Source: three-view drawing plus pictorial views. Frame: mm from the lowest corner of the part. A direction names the side the tool comes from. Give positions to 0.01 mm unless a question says otherwise; leave off trailing zeros. Loops run counter-clockwise (first coordinate to the right, second up) from the corner with the lowest first, then second, coordinate; pieces in that order, holes last. Notation, with made-up numbers: M -36,83.25 L -29,83.25 A18 ccw -29,114.25 Z; hole C 28.5,52.25 d8. An arc over 180 degrees is marked long. Write item = value, one per line.
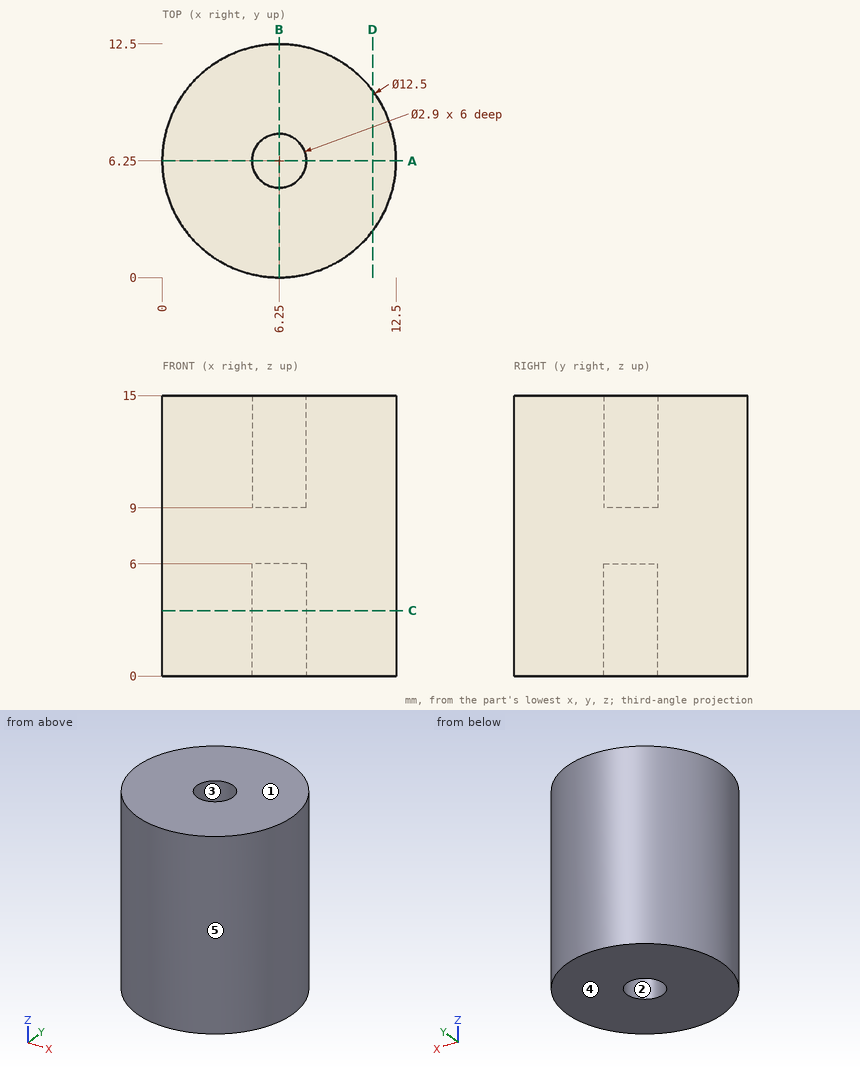
1. Cut plane C-C, the plane z = 3.5. Return the cut outline in (x, y), then the cut area to 3 significant figures.
Derived:
outline = C 6.25,6.25 d12.5; hole C 6.25,6.25 d2.9
area = 116 mm²
2. Material intervals for probe 1 along X at (y, z) = (6.25, 1.8); probe 2 along X at (y, z) = (4.25, 4.25), sorted ascending. Write a range as from..to.
Derived:
probe_1 = 0..4.8, 7.7..12.5
probe_2 = 0.33..12.17
3. Cut plane A-A, the plane y = 6.25. Return the cut outline in (x, z).
Derived:
outline = M 0,0 L 4.8,0 L 4.8,6 L 7.7,6 L 7.7,0 L 12.5,0 L 12.5,15 L 7.7,15 L 7.7,9 L 4.8,9 L 4.8,15 L 0,15 Z
4. Pull-direction query (X, two-part tool) for the marked faces 3, 4 and 5; classes: +X half, -X half, draft (parallel to the pull), parting line (faces both ways), or undercut.
Derived:
face_3 = undercut
face_4 = draft
face_5 = parting line
5. First-contact query: pin 1 Ø4.5 at (x, y) = (6.25, 6.25) entering from +Z; pin 2 Ø1.7 at (x, y) = (6.25, 6.25) entering from +Z; pin 3 Ø1.5 at (x, z) = (7.5, 12.5) entering from -Y; pin 4 Ø1.5 at (x, z) = (5, 2) entering from +Y. Flat tips, straight axial feed; report the tip coordinate or a pass-through.
Derived:
pin_1 = 15
pin_2 = 9
pin_3 = 0.02
pin_4 = 12.48
6. Reachability of the marked faces 1 and 2 from +Z, -Z, +X, -X, +Y, -Y: full face, straight path, thin tool, end or side. Return the list, or none.
Derived:
face_1 = +Z, +X, -X, +Y, -Y
face_2 = -Z
7. Cut plane D-D, the plane x = 11.25. Return the cut outline in (y, z), then the cut area to 4 significant figures.
Derived:
outline = M 2.5,0 L 10,0 L 10,15 L 2.5,15 Z
area = 112.5 mm²
